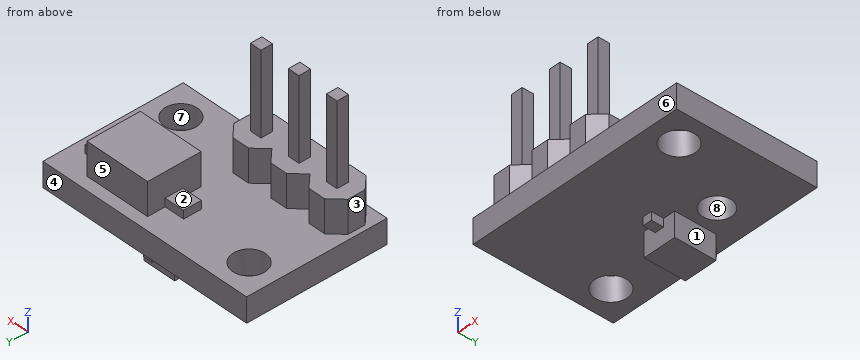
from build123d import *

# Parameters (mm, degrees)
SKETCH_W               = 13.6
SKETCH_H               = 8.6
PAD_DEPTH              = 1.5
SKETCH001_R            = 1
POCKET_DEPTH           = 5
SKETCH002_R            = 0.9
POCKET001_DEPTH        = 5
SKETCH003_W            = 4.055027
SKETCH003_H            = 3.273927
PAD001_DEPTH           = 2
SKETCH004_W            = 1.366968
SKETCH004_H            = 1.084461
PAD002_DEPTH           = 0.5
SKETCH005_W            = 2.05
SKETCH005_H            = 2.53
PAD003_DEPTH           = 1.5
SKETCH006_W            = 0.55793
SKETCH006_H            = 0.749967
PAD004_DEPTH           = 0.5
PAD005_DEPTH           = 2
SKETCH008_W            = 0.707107
SKETCH008_H            = 0.707107
PAD006_DEPTH           = 5
LINEARPATTERN_COUNT    = 3
LINEARPATTERN_PITCH    = 2.54
LINEARPATTERN001_COUNT = 3
LINEARPATTERN001_PITCH = 2.54


with BuildPart() as part:
    # Sketch → Pad (new body)
    with BuildSketch(Plane.XY):
        Rectangle(SKETCH_W, SKETCH_H)
    extrude(amount=PAD_DEPTH)

    # Sketch001 (on Face6 of Pad) → Pocket (cut)
    with BuildSketch(Plane.XY.offset(1.5)):
        with Locations((-5, 2.5)):
            Circle(SKETCH001_R)
        with Locations((5, -2.5)):
            Circle(SKETCH001_R)
    extrude(amount=-POCKET_DEPTH, mode=Mode.SUBTRACT)

    # Sketch002 (on Face4 of Pocket) → Pocket001 (cut)
    with BuildSketch(Plane(origin=(0, 0, 0), x_dir=(1, 0, 0), z_dir=(0, 0, -1))):
        with Locations((2.63, -1.991314)):
            Circle(SKETCH002_R)
    extrude(amount=-POCKET001_DEPTH, mode=Mode.SUBTRACT)

    # Sketch003 (on Face5 of Pocket001) → Pad001 (join)
    with BuildSketch(Plane.XY.offset(1.5)):
        with Locations((2.621891, 1.944408)):
            Rectangle(SKETCH003_W, SKETCH003_H)
    extrude(amount=PAD001_DEPTH)

    # Sketch004 (on Face5 of Pad001) → Pad002 (join)
    with BuildSketch(Plane.XY.offset(1.5)):
        with Locations((0.04648, 1.968005)):
            Rectangle(SKETCH004_W, SKETCH004_H)
        with Locations((5.259186, 1.968005)):
            Rectangle(SKETCH004_W, SKETCH004_H)
    extrude(amount=PAD002_DEPTH)

    # Sketch005 (on Face4 of Pad002) → Pad003 (join)
    with BuildSketch(Plane(origin=(0, 0, 0), x_dir=(1, 0, 0), z_dir=(0, 0, -1))):
        with Locations((0.15814, -2)):
            Rectangle(SKETCH005_W, SKETCH005_H)
    extrude(amount=PAD003_DEPTH)

    # Sketch006 (on Face4 of Pad003) → Pad004 (join)
    with BuildSketch(Plane(origin=(0, 0, 0), x_dir=(1, 0, 0), z_dir=(0, 0, -1))):
        with Locations((0.167423, -0.357102)):
            Rectangle(SKETCH006_W, SKETCH006_H)
        with Locations((0.167423, -3.601865)):
            Rectangle(SKETCH006_W, SKETCH006_H)
    extrude(amount=PAD004_DEPTH)

    # Sketch007 (on Face5 of Pad004) → Pad005 (join)
    with BuildSketch(Plane.XY.offset(1.5)):
        Polygon((-4.692553, -1.448605), (-5.744656, -1.448605), (-6.488605, -2.192553), (-6.488605, -3.244656), (-5.744656, -3.988605), (-4.692553, -3.988605), (-3.948605, -3.244656), (-3.948605, -2.192553), align=None)
    pad005 = extrude(amount=PAD005_DEPTH)

    # Sketch008 (on Face46 of Pad005) → Pad006 (join)
    with BuildSketch(Plane.XY.offset(3.5)):
        with Locations((-5.218604, -2.718604)):
            Rectangle(SKETCH008_W, SKETCH008_H)
    pad006 = extrude(amount=PAD006_DEPTH)

    # LinearPattern: Pad005 ×3
    with Locations(*[(i * LINEARPATTERN_PITCH, 0, 0) for i in range(1, LINEARPATTERN_COUNT)]):
        add(pad005)

    # LinearPattern001: Pad006 ×3
    with Locations(*[(i * LINEARPATTERN001_PITCH, 0, 0) for i in range(1, LINEARPATTERN001_COUNT)]):
        add(pad006)


solid = part.part
Can you work these out from the model? Positions are in its coordinate system, mm. Face numbers are marked on the shaded views. A direction names the side the tool comes from. Round coordinates to 2 decimals unless told otherwise and drop trailing zeros. Write each loop counter-clockwise with the first axis right and the second up, starting at its lowest first coordinate (ties: lowest second). Pieces come first, ordered by that corner, then holes. Notation, with made-up numbers: M -26.75,20.25 L 11.25,20.25 A19 cw 11.25,44.25 Z; hole C 54.5,87 d11. An arc over 180 degrees is marked long. Use a Markdown table: item, result.
Item 1: I want a section at B-B (x = 5). List the corners of the cut face in (y, z) for me, and give its area (3 significant figures).
Found:
| item | result |
|---|---|
| outline | M -4.3,0 L -3.5,0 L -3.5,1.5 L -4.3,1.5 Z; M -1.5,0 L 4.3,0 L 4.3,1.5 L 2.51,1.5 L 2.51,2 L 1.43,2 L 1.43,1.5 L -1.5,1.5 Z |
| area | 10.4 mm2 |
Item 2: Which directions (+Z, -Z, +X, -X, +Y, -Y) give clear straight access to the entire face, cutting with the end or side of a thin tool? Please do the marked faces 1, 2, 3 and 4.
Found:
| item | result |
|---|---|
| face 1 | -Z, +X, +Y, -Y |
| face 2 | +Z, -X, +Y |
| face 3 | +Z, -X, +Y, -Y |
| face 4 | +Z, -Z, +X, -X, +Y |
Item 3: I want a section at D-D (y = 1.75). List the corners of the cut face in (x, z) for me.
Found:
| item | result |
|---|---|
| outline | M -6.8,0 L -5.66,0 L -5.66,1.5 L -6.8,1.5 Z; M -4.34,0 L -0.87,0 L -0.87,-1.5 L 1.18,-1.5 L 1.18,0 L 1.76,0 L 1.76,1.5 L 3.5,1.5 L 3.5,0 L 6.8,0 L 6.8,1.5 L 5.94,1.5 L 5.94,2 L 4.65,2 L 4.65,3.5 L 0.59,3.5 L 0.59,2 L -0.64,2 L -0.64,1.5 L -4.34,1.5 Z |
Item 4: If I drill on line 1 along Y through (x, z) = (5, 0.9); line 2 along Y through (x, z) = (2.63, 0.95); line 3 along Z through (x, y) = (-1.25, 4), over which ranges is the centre line in solid material (lowest first)? Write a range as [from, to].
Found:
| item | result |
|---|---|
| line 1 | y = [-4.3, -3.5], [-1.5, 4.3] |
| line 2 | y = [-4.3, 1.09], [2.89, 4.3] |
| line 3 | z = [0, 1.5] |
Item 5: We'd pull the mould along Y, two halves only. Please class the marked faces 5, 6, 7 and 8: released by +Y, released by -Y, zero draft, split by the parting line, or undercut.
Found:
| item | result |
|---|---|
| face 5 | released by +Y |
| face 6 | released by -Y |
| face 7 | undercut |
| face 8 | undercut |
Item 6: For pin 1 Ø0.9 at (x, y) = (5.5, 2) entering from +Z; pin 2 Ø2 at (x, y) = (-2, 3) entering from -Z; pin 3 Ø4 at (x, z) = (-4.5, 4.5) entering from +Y, each with a flat end and sliding along its axis, tell me the tip position at first contact or that it passes through.
Found:
| item | result |
|---|---|
| pin 1 | stops at z = 2 |
| pin 2 | stops at z = 0 |
| pin 3 | stops at y = -1.45 |
Item 7: I want a section at C-C (z = 3). List the corners of the cut face in (x, y) for me.
Found:
| item | result |
|---|---|
| outline | M -6.49,-3.24 L -5.74,-3.99 L -4.69,-3.99 L -3.95,-3.24 L -3.2,-3.99 L -2.15,-3.99 L -1.41,-3.24 L -0.66,-3.99 L 0.39,-3.99 L 1.13,-3.24 L 1.13,-2.19 L 0.39,-1.45 L -0.66,-1.45 L -1.41,-2.19 L -2.15,-1.45 L -3.2,-1.45 L -3.95,-2.19 L -4.69,-1.45 L -5.74,-1.45 L -6.49,-2.19 Z; M 0.59,0.31 L 4.65,0.31 L 4.65,3.58 L 0.59,3.58 Z |
Item 8: I want a section at A-A (z = 5.25). List the corners of the cut face in (x, y) for me, and give its area (3 significant figures).
Found:
| item | result |
|---|---|
| outline | M -5.57,-3.07 L -4.87,-3.07 L -4.87,-2.37 L -5.57,-2.37 Z; M -3.03,-3.07 L -2.33,-3.07 L -2.33,-2.37 L -3.03,-2.37 Z; M -0.49,-3.07 L 0.21,-3.07 L 0.21,-2.37 L -0.49,-2.37 Z |
| area | 1.50 mm2 |
